Solid Edge part; units mm, degrees
sketch "Sketch1" plane through (0, 0, 0) normal (0, 0, 1) x (1, 0, 0)
  line L0 (-25, -57.5) -> (25, -57.5)
  line L1 (25, -57.5) -> (25, 57.5)
  line L2 (25, 57.5) -> (-25, 57.5)
  line L3 (-25, 57.5) -> (-25, -57.5)
  dimension "D1" = 25
  dimension "D2" = 25
extrude "Protrusion1" add sketch "Sketch1" along normal mid plane 6
fillet "Round_1" radius 5 4 edges at (25, 57.5, 0) (-25, 57.5, 0) (25, -57.5, 0) (-25, -57.5, 0)
hole "Hole_1" at (-20.5, 42.5, 3) direction (0, 0, -1) diameter 4.2 end up to next
hole "Hole1" at (20.5, 42.5, 3) direction (0, 0, -1) diameter 4.2 end up to next
hole "Hole_3" at (0, -45.5, -3) direction (0, 0, 1) diameter 6.6 end up to next countersink diameter 12 countersink angle 90
The model under review builds one solid part; all positions refer to its coordinate system, in mm. Round coordinates to 2 decimals unless told otherwise and drop trailing zeros. Loops run counter-clockwise (first coordinate to the right, second up) from the corner with the lowest first, then second, coordinate; pieces in that order, holes last.
1) Consider section D-D on y = 42.5. State the section outline as (x, z) points.
Values follow:
outline: (-25, -3) - (-22.6, -3) - (-22.6, 3) - (-25, 3) - close; (-18.4, -3) - (18.4, -3) - (18.4, 3) - (-18.4, 3) - close; (22.6, -3) - (25, -3) - (25, 3) - (22.6, 3) - close
2) The part is to be moulded in two halves that separate along X. For faces 1 (the face through (2.34, -48.06, -0.47)), 2 (the face through (25, -1, 0)), 3 (the face through (0, 1, -3)), say which applies: pulls with the +X half, pulls with the -X half, needs draft (parallel to the pull), parting line crosses it, or undercut.
Values follow:
face 1: undercut
face 2: pulls with the +X half
face 3: needs draft
3) Consider section A-A on x = 0. State the section outline as (y, z) points, then the cut area to 3 significant figures.
Values follow:
outline: (-57.5, -3) - (-51.5, -3) - (-48.8, -0.3) - (-48.8, 3) - (-57.5, 3) - close; (-42.2, -0.3) - (-39.5, -3) - (57.5, -3) - (57.5, 3) - (-42.2, 3) - close
area: 643 mm2
4) Consider section C-C on z = -1.3. State the section outline as (x, y) points.
Values follow:
outline: (-25, -52.5) arc R5 ccw to (-20, -57.5) - (20, -57.5) arc R5 ccw to (25, -52.5) - (25, 52.5) arc R5 ccw to (20, 57.5) - (-20, 57.5) arc R5 ccw to (-25, 52.5) - close; hole circle Ø4.2 at (-20.5, 42.5); hole circle Ø8.6 at (0, -45.5); hole circle Ø4.2 at (20.5, 42.5)
5) Consider section B-B on y = -45.5. State the section outline as (x, z) points, then the cut area to 3 significant figures.
Values follow:
outline: (-25, -3) - (-6, -3) - (-3.3, -0.3) - (-3.3, 3) - (-25, 3) - close; (3.3, -0.3) - (6, -3) - (25, -3) - (25, 3) - (3.3, 3) - close
area: 253 mm2
6) Wall thickness on line 1 along X through (y, z) = (42.5, 0.7); line 2 along Y through (x, z) = (-20.5, 1.4); line 3 along Y through (x, z) = (0, 2.25): over which ranges is each line inside the solid? List them lowest first.
Values follow:
line 1: x = -25 to -22.6, -18.4 to 18.4, 22.6 to 25
line 2: y = -57.47 to 40.4, 44.6 to 57.47
line 3: y = -57.5 to -48.8, -42.2 to 57.5
7) Clearance check with a flat-ended pin moving along its axis: P1, Ø10.5, axis at x = 0, y = -45.5, coming from the +Z side. State where the tip first meets the part, or that it passes through.
Values follow:
P1: stops at z = 3
